Geometry: see drawing. Coordinates: mm, zero at the bounding-box minimum. A direction names the side the tool comes from. Coordinates: 2 decimals unless noted, no trailing zeros. Order: outer loops, then holes, each group sorted by start corner. A loop starts at its lowest first (then second) coordinate and runs counter-clockwise, first axis right, second up.
Item 1: Contact query for flat-ended pins moving along their axis: P1, Ø1, axis at y = 11, z = 3, coming from the +X side; P2, Ø4.5, axis at x = 102, y = 19, coming from the +Z side; P3, Ø3, axis at x = 67.5, z = 6.5, coming from the +Y side. Output: stop coordinate, or through.
Item 2: Section A-A on y = 2.5. Return the cut outline in (x, z).
Item 3: Reachability of the marked faces 1 and 2 from +Z, -Z, +X, -X, +Y, -Y: full face, straight path, thin tool, end or side. Return the list, or none.
Item 4: Section D-D on z = 3. Return the cut outline in (x, y).
Item 5: Ray query, line 1 (X direction, y = 33.5, z = 0.3); line 2 (Y direction, x = 100.5, z = 1.15); line 3 (Y direction, x = 47, z = 3.5). Return the intervals inside material, ascending.
Item 6: Section B-B on y = 17.5. Return the cut outline in (x, z), then the cut area to 3 significant figures.
Item 7: Section C-C on x = 100.5. Return the cut outline in (y, z), then the cut area to 3 significant figures.
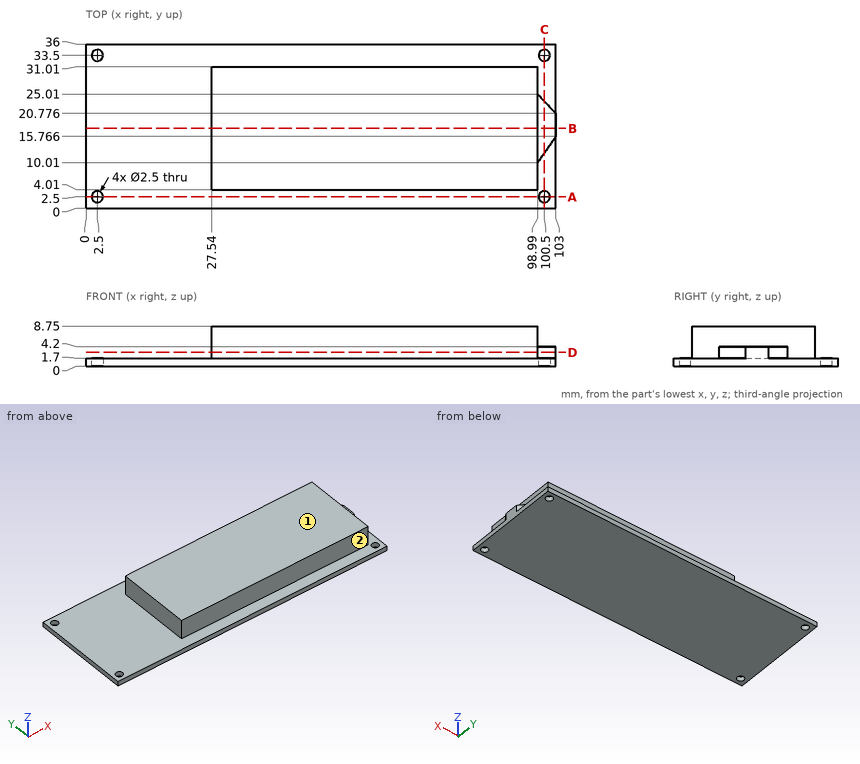
Answer list:
1. P1: stops at x = 100.03
1. P2: stops at z = 4.2
1. P3: stops at y = 31.01
2. outline: (0, 0) - (1.25, 0) - (1.25, 1.7) - (0, 1.7) - close; (3.75, 0) - (99.25, 0) - (99.25, 1.7) - (3.75, 1.7) - close; (101.75, 0) - (103, 0) - (103, 1.7) - (101.75, 1.7) - close
3. face 1: +Z, +X, -X, +Y, -Y
3. face 2: +Z, +X, -X, -Y
4. outline: (27.54, 4.01) - (98.99, 4.01) - (98.99, 10.01) - (103, 15.77) - (103, 20.78) - (98.99, 25.01) - (98.99, 31.01) - (27.54, 31.01) - close
5. line 1: x = 0 to 1.25, 3.75 to 99.25, 101.75 to 103
5. line 2: y = 0 to 1.25, 3.75 to 32.25, 34.75 to 36
5. line 3: y = 4.01 to 31.01
6. outline: (0, 0) - (103, 0) - (103, 4.2) - (98.99, 4.2) - (98.99, 8.75) - (27.54, 8.75) - (27.54, 1.7) - (0, 1.7) - close
6. area: 689 mm2
7. outline: (0, 0) - (1.25, 0) - (1.25, 1.7) - (0, 1.7) - close; (3.75, 0) - (32.25, 0) - (32.25, 1.7) - (23.42, 1.7) - (23.42, 4.2) - (12.18, 4.2) - (12.18, 1.7) - (3.75, 1.7) - close; (34.75, 0) - (36, 0) - (36, 1.7) - (34.75, 1.7) - close
7. area: 80.8 mm2
